Input: part model. Units: mm. Frame: model coordinates. Face numbers are marked on the shaded views. A direction names the side the tool comes from. Coordinates: 2 decimals unless noted, no trailing zeros. Write each loop counter-clockwise with the first axis right and the second up, starting at its lowest first coordinate (ties: lowest second). Pieces come first, ordered by that corner, then holes. Notation, with made-up numbers: (-5.5, 32) - (15.5, 32) arc R24 cw to (15.5, 63) - close; hole circle Ø8 at (57, -32.5). An arc over 180 degrees is marked (long way). Use a Markdown table: item, result. Add a question column.
Q1. Set-up query: the marked faces 1 and 2. Return all of +Z, -Z, +X, -X, +Y, -Y with unobstructed straight access to the full face (end or side cutting, diameter ignored); none if empty.
Q2. Section query B-B (z = 19.75). Return the cut outline in (x, y).
Q3. Section query A-A (x = 21.5). Return the cut outline in (y, z).
Q4. Section query C-C (y = 2.7). Return the cut outline in (x, z), then the cut area to 3 significant figures.
Q5. Pin query (flat end, axial travel): P1, Ø1, axis at x = 21, y = 4, coming from the -Z side. Return the tip coordinate at first contact, or that it passes through.
Q6. Section query D-D (x = 25.75). Return the cut outline in (y, z), then the cut area to 4 significant figures.
Q7. Material intervals for probe 1 along Y at (x, z) = (22.25, 22); probe 2 along X at (y, z) = (4.85, 19.75); probe 3 along X at (y, z) = (4.6, 19), sorted ascending. Write a range as from..to.
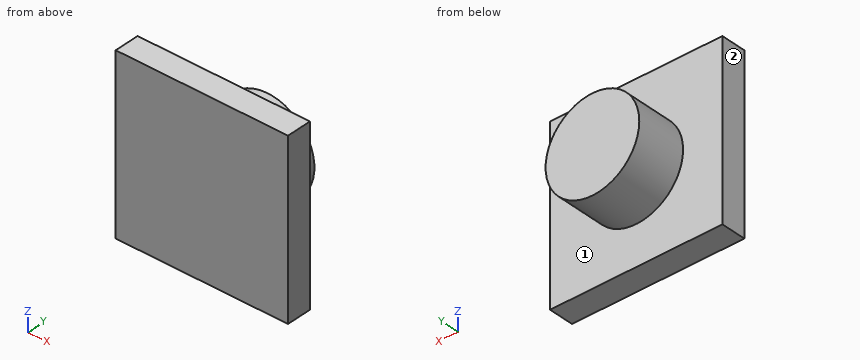
Autodesk Fusion 360 part; units mm, degrees
sketch "Schizzo1" plane through (0, 0, 0) normal (0, 1, 0) x (1, 0, 0)
  line L0 (19.547, -15.8464) -> (25.847, -15.8464)
  line L1 (25.847, -15.8464) -> (25.847, -22.1464)
  line L2 (25.847, -22.1464) -> (19.547, -22.1464)
  line L3 (19.547, -22.1464) -> (19.547, -15.8464)
  line L4 (27.847, -24.1464) -> (17.547, -24.1464)
  line L5 (17.547, -24.1464) -> (17.547, -13.8464)
  line L6 (17.547, -13.8464) -> (27.847, -13.8464)
  line L7 (27.847, -13.8464) -> (27.847, -24.1464)
  dimension "d1" = 6.3
  dimension "d2" = 6.3
  dimension "d3" = -2
extrude "Estrusione1" add sketch "Schizzo1" along normal blind 2 contours L0 L1 L2 L3 | L4 L5 L6 L7
extrude "Estrusione2" add sketch "Schizzo1" along normal blind 7 contours L0 L1 L2 L3
extrude "Estrusione3" cut 1 faces at (21.647, 7, 17.9464) along direction (0, -1, 0) blind 2
move_face "FacceDiOffset1" offset -0.15 4 faces at (21.647, 3, 15.8464) (19.547, 3, 20.0464) (23.747, 3, 22.1464) (25.847, 3, 17.9464)
extrude "Estrusione4" cut 1 faces at (25.697, 4, 19.9964) along direction (-1, 0, 0) blind 0.2
extrude "Estrusione5" cut 1 faces at (23.5637, 3, 15.9964) along direction (0, 0, 1) blind 0.2
extrude "Estrusione6" cut 1 faces at (19.697, 3, 20.063) along direction (1, 0, 0) blind 0.2
extrude "Estrusione7" cut 1 faces at (23.6304, 4, 21.9964) along direction (0, 0, -1) blind 0.2
extrude "Estrusione8" cut 1 faces at (24.4137, 0, 17.2797) along direction (0, 1, 0) blind 0.5
sketch "Schizzo2" plane through (0, 5, 0) normal (0, 1, 0) x (-1, 0, 0)
  line L0 (-19.897, 21.7964) -> (-25.497, 21.7964)
  line L1 (-25.497, 21.7964) -> (-25.497, 16.1964)
  line L2 (-25.497, 16.1964) -> (-19.897, 16.1964)
  line L3 (-19.897, 16.1964) -> (-19.897, 21.7964)
  circle A0 centre (-22.697, 18.9964) radius 2.8
extrude "Estrusione9" cut sketch "Schizzo2" against normal blind 3 contours L0 L3 A0 | L0 L1 A0 | L2 L3 A0 | L1 L2 A0
Values follow:
| question | item | result |
|---|---|---|
| 1 | face 1 | +Y |
| 1 | face 2 | +Z, -Z, -X, +Y, -Y |
| 2 | outline | (17.55, 0.5) - (27.85, 0.5) - (27.85, 2) - (25.39, 2) - (25.39, 5) - (20, 5) - (20, 2) - (17.55, 2) - close |
| 3 | outline | (0.5, 13.85) - (2, 13.85) - (2, 16.47) - (5, 16.47) - (5, 21.53) - (2, 21.53) - (2, 24.15) - (0.5, 24.15) - close |
| 4 | outline | circle Ø5.6 at (22.7, 19) |
| 4 | area | 24.6 mm2 |
| 5 | P1 | z = 16.47 |
| 6 | outline | (0.5, 13.85) - (2, 13.85) - (2, 24.15) - (0.5, 24.15) - close |
| 6 | area | 15.45 mm2 |
| 7 | probe 1 | 0.5..2 |
| 7 | probe 2 | 20..25.39 |
| 7 | probe 3 | 19.9..25.5 |
